Work out the finished part from the listing and answer in its coordinate system (mm). A direction names the side the tool comes from. Give positions to 0.01 mm unless a question says otherwise; leave off trailing zeros. Loops run counter-clockwise (first coordinate to the right, second up) from the corner with the lowest first, then second, coordinate; pieces in that order, holes last. Notation, with made-up numbers: (42.25, -32.5) -> (93.25, -32.5) arc R35 ccw to (93.25, 1.5) -> close; hole circle Ø1 at (48, 27). An arc over 180 degrees is marked (long way). Answer as CSV lines item,"result". Start each with the question number.
1. Determine the mould class of faces 3 (the face through (12.4, -50, -4)), 4 (the face through (8.767, -55.07, -16.856)), 5 (the face through (0, 0, 0)) for opening direction Y: +Y half, -Y half, draft (parallel to the pull), parting line (faces both ways), or undercut.
2. Find section C-C, the plane z = 10.5. Give the vertices of the cut face in (x, y).
3. Find section B-B, the plane x = 0. Give the vertices of the cut face in (y, z), and give its area (3 significant figures).
4. Flat-ended cylindrical pins translate along their axes: pin 1 Ø3 at (y, z) = (-21.5, -5) entering from -X; pin 2 Ø3 at (x, y) = (-8.5, -28.5) entering from -Z; pin 3 Ø6 at (y, z) = (-10.5, -6.5) entering from +X; pin 4 Ø5 at (x, z) = (5.5, -15) entering from +Y. Find the tip coordinate at first contact, or state that the pin passes through.
5. Find section A-A, the plane x = -17. Give the vertices of the cut face in (y, z).
6. A tool of negligible diameter and unlimited length cuts with its end or side. For faces 1 (the face through (11.923, -29.72, 3.755)), 2 (the face through (0, -60, 0)), from which of +Z, -Z, +X, -X, +Y, -Y can it reach the whole face along a straight path? Write none if from no direction.
7. Find section D-D, the plane y = -29. Give the vertices of the cut face in (x, z).
8. Find the intervals of material crossed by line 1 along Y through (x, z) = (10, -10); line 2 along X through (y, z) = (-24.5, -0.5); line 3 along X through (y, z) = (-17.5, 3), in increasing order.
from build123d import *

# Parameters (mm, degrees)
SKETCH1_R           = 19
BOSS_EXTRUDE1_DEPTH = 10
SKETCH2_R           = 12.5
BOSS_EXTRUDE2_DEPTH = 50
SKETCH4_R           = 19
BOSS_EXTRUDE3_DEPTH = 10


with BuildPart() as part:
    # Sketch1 → Boss-Extrude1 (new body)
    with BuildSketch(Plane(origin=(0, 0, 0), x_dir=(1, 0, 0), z_dir=(0, 1, 0))):
        Circle(SKETCH1_R)
    extrude(amount=-BOSS_EXTRUDE1_DEPTH)

    # Sketch2 → Boss-Extrude2 (add)
    with BuildSketch(Plane.XZ.offset(10)):
        Circle(SKETCH2_R)
    extrude(amount=BOSS_EXTRUDE2_DEPTH)

    # Sketch4 → Boss-Extrude3 (add)
    with BuildSketch(Plane.XZ.offset(60)):
        Circle(SKETCH4_R)
    extrude(amount=-BOSS_EXTRUDE3_DEPTH)


solid = part.part
Resolved:
1,face 3,"undercut"
1,face 4,"draft"
1,face 5,"+Y half"
2,outline,"(-15.84, -60) -> (15.84, -60) -> (15.84, -50) -> (6.78, -50) -> (6.78, -10) -> (15.84, -10) -> (15.84, 0) -> (-15.84, 0) -> (-15.84, -10) -> (-6.78, -10) -> (-6.78, -50) -> (-15.84, -50) -> close"
3,outline,"(-60, -19) -> (-50, -19) -> (-50, -12.5) -> (-10, -12.5) -> (-10, -19) -> (0, -19) -> (0, 19) -> (-10, 19) -> (-10, 12.5) -> (-50, 12.5) -> (-50, 19) -> (-60, 19) -> close"
3,area,"1,760 mm^2"
4,pin 1,"stops at x = -12"
4,pin 2,"stops at z = -10.36"
4,pin 3,"stops at x = 18.67"
4,pin 4,"stops at y = 0"
5,outline,"(-60, -8.49) -> (-50, -8.49) -> (-50, 8.49) -> (-60, 8.49) -> close; (-10, -8.49) -> (0, -8.49) -> (0, 8.49) -> (-10, 8.49) -> close"
6,face 1,"none"
6,face 2,"+Z, -Z, +X, -X, -Y"
7,outline,"circle Ø25 at (0, 0)"
8,line 1,"y = -60 to -50, -10 to 0"
8,line 2,"x = -12.49 to 12.49"
8,line 3,"x = -12.13 to 12.13"
